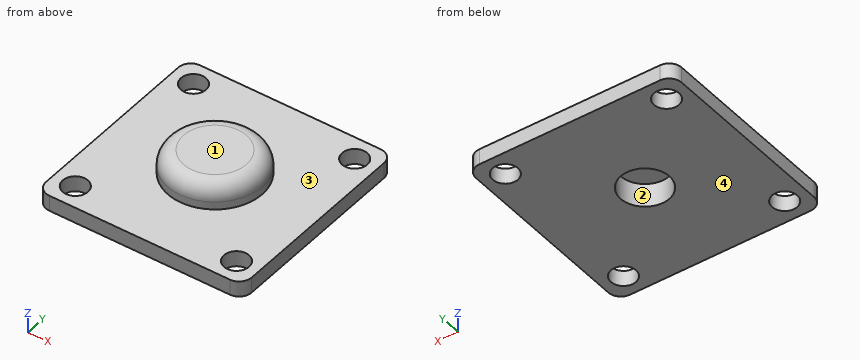
from build123d import *

# Parameters (mm, degrees)
SKETCH_1_W          = 26.162950904
SKETCH_1_H          = 26.162950904
SKETCH_1_R          = 1.6
EXTRUDE_1_DEPTH     = 2
SKETCH_2_R          = 6
EXTRUDE_2_DEPTH     = 3
SKETCH_3_R          = 3.1
CUT_EXTRUDE_1_DEPTH = 3
FILLET_2_R          = 2
FILLET_3_R          = 1.6


with BuildPart() as part:
    # 草图1 → 凸台-拉伸1 (new body)
    with BuildSketch(Plane.XY):
        Rectangle(SKETCH_1_W, SKETCH_1_H)
        with Locations((10.253048327, 10.253048327)):
            Circle(SKETCH_1_R, mode=Mode.SUBTRACT)
        with Locations((-10.253048327, 10.253048327)):
            Circle(SKETCH_1_R, mode=Mode.SUBTRACT)
        with Locations((-10.253048327, -10.253048327)):
            Circle(SKETCH_1_R, mode=Mode.SUBTRACT)
        with Locations((10.253048327, -10.253048327)):
            Circle(SKETCH_1_R, mode=Mode.SUBTRACT)
    extrude(amount=EXTRUDE_1_DEPTH)

    # 草图2 → 凸台-拉伸2 (add)
    with BuildSketch(Plane.XY.offset(2)):
        Circle(SKETCH_2_R)
    extrude(amount=EXTRUDE_2_DEPTH)

    # 草图3 → 切除-拉伸1 (cut)
    with BuildSketch(Plane(origin=(0, 0, 0), x_dir=(-1, 0, 0), z_dir=(0, 0, -1))):
        Circle(SKETCH_3_R)
    extrude(amount=-CUT_EXTRUDE_1_DEPTH, mode=Mode.SUBTRACT)

    # 圆角2
    fillet_2_edges = [part.edges().sort_by_distance(p)[0] for p in [
        (-6, 0, 5),
    ]]
    fillet(fillet_2_edges, radius=FILLET_2_R)

    # 圆角3
    fillet_3_edges = [part.edges().sort_by_distance(p)[0] for p in [
        (13.081475452, -13.081475452, 1),
        (-13.081475452, -13.081475452, 1),
        (-13.081475452, 13.081475452, 1),
        (13.081475452, 13.081475452, 1),
    ]]
    fillet(fillet_3_edges, radius=FILLET_3_R)


solid = part.part
Design review of the part built by this model. Coordinates are the model's own, in mm. Face numbers are marked on the shaded views. A direction names the side the tool comes from. Give positions to 0.01 mm unless a question says otherwise; leave off trailing zeros. Loops run counter-clockwise (first coordinate to the right, second up) from the corner with the lowest first, then second, coordinate; pieces in that order, holes last. Notation, with made-up numbers: M 51,53 L 92,53 A8 ccw 92,63 Z; hole C 64.25,80 d7. An arc over 180 degrees is marked long. Write item = value, one per line.
Q1. We need section C-C (z = 2.4). Give the boundary of the cut face in (x, y).
Output values:
outline = C 0,0 d12; hole C 0,0 d6.2
Q2. We need section D-D (y = -7.75). Give the boundary of the cut face in (x, z).
Output values:
outline = M -13.08,0 L 13.08,0 L 13.08,2 L -13.08,2 Z
Q3. Draft analysis for pull direction Y (two halves, no side actions). For the marked faces 1 and 2, state which applies: +Y half, -Y half, draft (parallel to the pull), parting line (faces both ways), or undercut.
Output values:
face_1 = draft
face_2 = undercut
Q4. We need section A-A (x = 0). Give the boundary of the cut face in (y, z).
Output values:
outline = M -13.08,0 L -3.1,0 L -3.1,3 L 3.1,3 L 3.1,0 L 13.08,0 L 13.08,2 L 6,2 L 6,3 A2 ccw 4,5 L -4,5 A2 ccw -6,3 L -6,2 L -13.08,2 Z
Q5. For the marked faces 3 and 4, list the 3-axis set-ups (+Z, -Z, +X, -X, +Y, -Y) from which the entire face can be reached by the end or side of a thin tool; tool diameter is ignored.
Output values:
face_3 = +Z
face_4 = -Z, +X, -X, +Y, -Y
Q6. Insertion check: pin 1 (12 mm diameter, centred on x = -8, y = 8.5, fed in from +Z); pin 2 (10 mm diameter, centred on x = 7, y = -6, fed in from +Z); pin 3 (5 mm diameter, centred on x = 10.25, y = -10.25, fed in from +Z). Each pin has a flat end and moves straight along its axis. Give the tip position at first contact, or say it passes through.
Output values:
pin_1 = 4.1
pin_2 = 4.99
pin_3 = 2
Q7. We need section B-B (x = 9.5). Give the boundary of the cut face in (y, z), plus the area to 3 significant figures.
Output values:
outline = M -13.08,0 L -11.66,0 L -11.66,2 L -13.08,2 Z; M -8.84,0 L 8.84,0 L 8.84,2 L -8.84,2 Z; M 11.66,0 L 13.08,0 L 13.08,2 L 11.66,2 Z
area = 41.0 mm^2
Q8. To check wall thickness, follow line 1 (Z direction, x = -9.5, y = 3.5); line 2 (X direction, y = -9.5, z = 0.9); line 3 (Y direction, x = -1.75, z = 1.85). State the ranges of each line that lie inside material, in increasing order. Write a range as [from, to].
Output values:
line_1 = [0, 2]
line_2 = [-13.08, -11.66], [-8.84, 8.84], [11.66, 13.08]
line_3 = [-13.08, -2.56], [2.56, 13.08]
